from build123d import *

# Parameters (mm, degrees)
F0_W      = 63.5
F0_H      = 44.45
F1_DEPTH  = 38.1
F2_W      = 25.4
F2_H      = 38.1
F3_DEPTH  = 63.501
F4_W      = 25.4
F4_H      = 38.1
F5_DEPTH  = 12.701
F7_DEPTH  = 12.701
F8_R      = 6.35
F9_DEPTH  = 12.701
F11_DEPTH = 12.701
F13_DEPTH = 12.701
F15_DEPTH = 25.4
F17_DEPTH = 6.351


with BuildPart() as f1:
    # F0 (on Front) → F1 (new body)
    with BuildSketch(Plane.XZ):
        with Locations((-31.75, 22.225)):
            Rectangle(F0_W, F0_H)
    extrude(amount=F1_DEPTH)

    # F2 (on face) → F3 (cut, through all)
    with BuildSketch(Plane(origin=(-63.5, 0, 0), x_dir=(0, -1, 0), z_dir=(-1, 0, 0))):
        with Locations((25.4, 25.4)):
            Rectangle(F2_W, F2_H)
    extrude(amount=-F3_DEPTH, mode=Mode.SUBTRACT)

    # F4 (on face) → F5 (cut, through all)
    with BuildSketch(Plane.XZ.offset(12.7)):
        with Locations((-12.7, 25.4)):
            Rectangle(F4_W, F4_H)
    extrude(amount=-F5_DEPTH, mode=Mode.SUBTRACT)

    # F6 (on face) → F7 (cut, through all)
    with BuildSketch(Plane.XZ.offset(12.7)):
        with BuildLine():
            Line((-38.1, 44.45), (-50.8, 44.45))
            ThreePointArc((-50.8, 44.45), (-41.8197438789, 40.7302561211), (-38.1, 31.75))
            Line((-38.1, 31.75), (-38.1, 44.45))
        make_face()
        with BuildLine():
            Line((-50.8, 44.45), (-63.5, 44.45))
            Line((-63.5, 44.45), (-63.5, 31.75))
            ThreePointArc((-63.5, 31.75), (-59.7802561211, 40.7302561211), (-50.8, 44.45))
        make_face()
    extrude(amount=-F7_DEPTH, mode=Mode.SUBTRACT)

    # F8 (on face) → F9 (cut, through all)
    with BuildSketch(Plane.XZ.offset(12.7)):
        with Locations((-50.8, 31.75)):
            Circle(F8_R)
    extrude(amount=-F9_DEPTH, mode=Mode.SUBTRACT)

    # F10 (on face) → F11 (cut, through all)
    with BuildSketch(Plane.XZ.offset(12.7)):
        Polygon((-38.1, 44.45), (-38.1, 31.75), (-38.1, 19.05), (-25.4, 19.05), (-25.4, 44.45), align=None)
    extrude(amount=-F11_DEPTH, mode=Mode.SUBTRACT)

    # F12 (on face) → F13 (cut, through all)
    with BuildSketch(Plane.XZ.offset(12.7)):
        with BuildLine():
            Line((-25.4, 19.05), (-38.1, 19.05))
            ThreePointArc((-38.1, 19.05), (-34.3802561211, 10.0697438789), (-25.4, 6.35))
            Line((-25.4, 6.35), (-25.4, 19.05))
        make_face()
    extrude(amount=-F13_DEPTH, mode=Mode.SUBTRACT)

    # F14 (on face) → F15 (cut)
    with BuildSketch(Plane.XY.offset(6.35)):
        with BuildLine():
            Line((-63.5, -31.75), (-63.5, -38.1))
            Line((-63.5, -38.1), (-57.15, -38.1))
            ThreePointArc((-57.15, -38.1), (-61.6401280605, -36.2401280605), (-63.5, -31.75))
        make_face()
    extrude(amount=-F15_DEPTH, mode=Mode.SUBTRACT)

    # F16 (on face) → F17 (cut, through all)
    with BuildSketch(Plane.XY.offset(6.35)):
        with BuildLine():
            Line((-6.35, -38.1), (0, -38.1))
            Line((0, -38.1), (0, -31.75))
            ThreePointArc((0, -31.75), (-1.8598719395, -36.2401280605), (-6.35, -38.1))
        make_face()
    extrude(amount=-F17_DEPTH, mode=Mode.SUBTRACT)


solid = f1.part
Design review of the part built by this model. Coordinates are the model's own, in mm. A direction names the side the tool comes from. Coordinates: 2 decimals unless noted, no trailing zeros. Write each loop counter-clockwise with the first axis right and the second up, starting at its lowest first coordinate (ties: lowest second). Pieces come first, ordered by that corner, then holes. Notation, with made-up numbers: (42.25, 11) - (65.25, 11) arc R38 ccw to (65.25, 50) - close; hole circle Ø2 at (28.5, -20). An arc over 180 degrees is marked (long way). One line per item, written item: value.
1) Mouldability with a two-part tool opening along X and no side actions: class faces 3 (the face through (-49, -12.7, 25)), 4 (the face through (-38.1, -6, 25)), 5 (the face through (-44.743, -6.439, 33.657)) as +X half, -X half, draft (parallel to the pull), parting line (faces both ways), or undercut.
Answer sheet:
face 3: draft
face 4: +X half
face 5: undercut
2) Add section A-A (y = -4). State the section outline as (x, z) points, plus the area to 3 significant figures.
Answer sheet:
outline: (-63.5, 0) - (0, 0) - (0, 6.35) - (-25.4, 6.35) arc R12.7 cw to (-38.1, 19.05) - (-38.1, 31.75) arc R12.7 ccw to (-63.5, 31.75) - close; hole circle Ø12.7 at (-50.8, 31.75)
area: 1,210 mm2
3) Insertion check: pin 1 (4 mm diameter, centred on y = -6, z = 23.5, fed in from +X); pin 2 (14.5 mm diameter, centred on x = -50.8, z = 31.75, fed in from -Y); pin 3 (3 mm diameter, centred on x = -33, y = -14.5, fed in from +Z). Each pin has a flat end and moves straight along its axis. Give the tip position at first contact, or say it passes through.
Answer sheet:
pin 1: stops at x = -38.1
pin 2: stops at y = -12.7
pin 3: stops at z = 6.35
4) Add section D-D (x = -11.5). State the section outline as (y, z) points, plus the area to 3 significant figures.
Answer sheet:
outline: (-38.1, 0) - (0, 0) - (0, 6.35) - (-38.1, 6.35) - close
area: 242 mm2
5) To check wall thickness, follow probe 1 along Z at (x, y) = (-50.8, -8.5); probe 2 along Z at (x, y) = (-24.5, -36); probe 3 along Y at (x, z) = (-58.5, 24). State the ranges of each line that lie inside material, in increasing order.
Answer sheet:
probe 1: z = 0 to 25.4, 38.1 to 44.45
probe 2: z = 0 to 6.35
probe 3: y = -12.7 to 0
6) For faces 1 (the face through (-61.59, -36.29, 3.22)), 2 (the face through (-32, -23, 6.35)), list the 3-axis set-ups (+Z, -Z, +X, -X, +Y, -Y) from which the entire face can be reached by the end or side of a thin tool; tool diameter is ignored.
Answer sheet:
face 1: +Z, -Z, -X, -Y
face 2: +Z, +X, -Y
7) Add section B-B (z = 32.5). State the section outline as (x, y) points, plus the area to 3 significant figures.
Answer sheet:
outline: (-63.48, -12.7) - (-57.11, -12.7) - (-57.11, 0) - (-63.48, 0) - close; (-44.49, -12.7) - (-38.12, -12.7) - (-38.12, 0) - (-44.49, 0) - close
area: 162 mm2
8) Add section C-C (y = -21). State the section outline as (x, z) points.
Answer sheet:
outline: (-63.5, 0) - (0, 0) - (0, 6.35) - (-63.5, 6.35) - close
